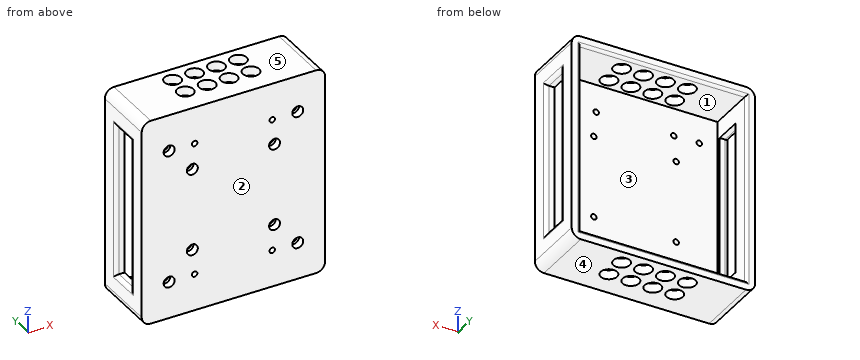
```python
from build123d import *

# Parameters (mm, degrees)
SKETCH1_W            = 100.4
SKETCH1_H            = 113.4
BOSS_EXTRUDE2_DEPTH  = 35
SKETCH2_W            = 90.4
SKETCH2_H            = 103.4
CUT_EXTRUDE1_DEPTH   = 27
FILLET4_R            = 5
SKETCH4_W            = 83.4
SKETCH4_H            = 15
CUT_EXTRUDE3_DEPTH   = 123
FILLET5_R            = 2
FILLET6_R            = 2
SKETCH3_R            = 4.5
CUT_EXTRUDE4_DEPTH   = 123
SKETCH5_R            = 1.5
CUT_EXTRUDE5_DEPTH   = 37
SKETCH6_R            = 3
CUT_EXTRUDE6_DEPTH   = 4
SKETCH7_R            = 1.5
CUT_EXTRUDE7_DEPTH   = 17
SKETCH8_R            = 1.5
CUT_EXTRUDE8_DEPTH   = 9
SKETCH9_R            = 3
CUT_EXTRUDE9_DEPTH   = 4
LPATTERN2_COUNT      = 4
LPATTERN2_PITCH      = 12
LPATTERN2_COUNT_DIR2 = 2
LPATTERN2_PITCH_DIR2 = 12
FILLET7_R            = 1.5


with BuildPart() as part:
    # Sketch1 → Boss-Extrude2 (new body)
    with BuildSketch(Plane(origin=(0, 0, 0), x_dir=(1, 0, 0), z_dir=(0, 1, 0))):
        Rectangle(SKETCH1_W, SKETCH1_H)
    extrude(amount=BOSS_EXTRUDE2_DEPTH)

    # Sketch2 → Cut-Extrude1 (cut)
    with BuildSketch(Plane(origin=(0, 35, 0), x_dir=(1, 0, 0), z_dir=(0, 1, 0))):
        Rectangle(SKETCH2_W, SKETCH2_H)
    extrude(amount=-CUT_EXTRUDE1_DEPTH, mode=Mode.SUBTRACT)

    # Fillet4
    fillet4_edges = [part.edges().sort_by_distance(p)[0] for p in [
        (-50.2, 17.5, 56.7),
        (50.2, 17.5, 56.7),
        (50.2, 17.5, -56.7),
        (-50.2, 17.5, -56.7),
    ]]
    fillet(fillet4_edges, radius=FILLET4_R)

    # Sketch4 → Cut-Extrude3 (cut)
    with BuildSketch(Plane(origin=(50.2, 0, 0), x_dir=(0, 0, -1), z_dir=(1, 0, 0))):
        with Locations((0, 17.5)):
            Rectangle(SKETCH4_W, SKETCH4_H)
    extrude(amount=-CUT_EXTRUDE3_DEPTH, mode=Mode.SUBTRACT)

    # Fillet5
    fillet5_edges = [part.edges().sort_by_distance(p)[0] for p in [
        (50.2, 17.5, 41.7),
        (50.2, 10, 0),
        (50.2, 17.5, -41.7),
        (50.2, 25, 0),
    ]]
    fillet(fillet5_edges, radius=FILLET5_R)

    # Fillet6
    fillet6_edges = [part.edges().sort_by_distance(p)[0] for p in [
        (-50.2, 17.5, 41.7),
        (-50.2, 25, 0),
        (-50.2, 17.5, -41.7),
        (-50.2, 10, 0),
    ]]
    fillet(fillet6_edges, radius=FILLET6_R)

    # Sketch3 → Cut-Extrude4 (cut)
    with BuildSketch(Plane(origin=(0, 0, -56.7), x_dir=(-1, 0, 0), z_dir=(0, 0, -1))):
        with Locations((-18, 14.5)):
            Circle(SKETCH3_R)
    cut_extrude4 = extrude(amount=-CUT_EXTRUDE4_DEPTH, mode=Mode.SUBTRACT)

    # Sketch5 → Cut-Extrude5 (cut)
    with BuildSketch(Plane(origin=(0, 8, 0), x_dir=(1, 0, 0), z_dir=(0, 1, 0))):
        with Locations((-22.5, 22.5)):
            Circle(SKETCH5_R)
        with Locations((22.5, 22.5)):
            Circle(SKETCH5_R)
        with Locations((-22.5, -22.5)):
            Circle(SKETCH5_R)
        with Locations((22.5, -22.5)):
            Circle(SKETCH5_R)
    extrude(amount=-CUT_EXTRUDE5_DEPTH, mode=Mode.SUBTRACT)

    # Sketch6 → Cut-Extrude6 (cut)
    with BuildSketch(Plane.XZ):
        with Locations((-22.5, 22.5)):
            Circle(SKETCH6_R)
        with Locations((-22.5, -22.5)):
            Circle(SKETCH6_R)
        with Locations((22.5, 22.5)):
            Circle(SKETCH6_R)
        with Locations((22.5, -22.5)):
            Circle(SKETCH6_R)
    extrude(amount=-CUT_EXTRUDE6_DEPTH, mode=Mode.SUBTRACT)

    # Sketch7 → Cut-Extrude7 (cut)
    with BuildSketch(Plane.XZ):
        with Locations((-21.25, 36.5)):
            Circle(SKETCH7_R)
        with Locations((-21.25, -36.5)):
            Circle(SKETCH7_R)
        with Locations((21.25, -36.5)):
            Circle(SKETCH7_R)
        with Locations((21.25, 36.5)):
            Circle(SKETCH7_R)
    extrude(amount=-CUT_EXTRUDE7_DEPTH, mode=Mode.SUBTRACT)

    # Sketch8 → Cut-Extrude8 (cut)
    with BuildSketch(Plane(origin=(0, 8, 0), x_dir=(1, 0, 0), z_dir=(0, 1, 0))):
        with Locations((-35.2, 36.6)):
            Circle(SKETCH8_R)
        with Locations((35.2, 36.6)):
            Circle(SKETCH8_R)
        with Locations((-35.2, -36.7)):
            Circle(SKETCH8_R)
        with Locations((35.2, -36.7)):
            Circle(SKETCH8_R)
    extrude(amount=-CUT_EXTRUDE8_DEPTH, mode=Mode.SUBTRACT)

    # Sketch9 → Cut-Extrude9 (cut)
    with BuildSketch(Plane.XZ):
        with Locations((-35.2, 36.7)):
            Circle(SKETCH9_R)
        with Locations((35.2, 36.7)):
            Circle(SKETCH9_R)
        with Locations((-35.2, -36.6)):
            Circle(SKETCH9_R)
        with Locations((35.2, -36.6)):
            Circle(SKETCH9_R)
    extrude(amount=-CUT_EXTRUDE9_DEPTH, mode=Mode.SUBTRACT)

    # LPattern2: Cut-Extrude4 4 × 2
    with Locations(*[(-i * LPATTERN2_PITCH, j * LPATTERN2_PITCH_DIR2, 0) for i in range(LPATTERN2_COUNT) for j in range(LPATTERN2_COUNT_DIR2) if (i, j) != (0, 0)]):
        add(cut_extrude4, mode=Mode.SUBTRACT)

    # Fillet7
    fillet7_edges = [part.edges().sort_by_distance(p)[0] for p in [
        (45.2, 35, 0),
        (0, 35, -51.7),
        (-45.2, 35, 0),
        (0, 35, 51.7),
    ]]
    fillet(fillet7_edges, radius=FILLET7_R)


solid = part.part
```
Check sheet for the modelled part. Datum: model origin and axes. Units: mm. Face numbers are marked on the shaded views. A direction names the side the tool comes from. Give positions to 0.01 mm unless a question says otherwise; leave off trailing zeros. Write each loop counter-clockwise with the first axis right and the second up, starting at its lowest first coordinate (ties: lowest second). Pieces come first, ordered by that corner, then holes.
Item 1: Gauge pin test, flat ends, axial feed: pin 1 (10 mm diameter, centred on y = 16, z = -43, fed in from -X); pin 2 (0.9 mm diameter, centred on x = 46, z = -20, fed in from +Y); pin 3 (1.5 mm diameter, centred on x = -47, y = 16.5, fed in from +Z); pin 4 (5.5 mm diameter, centred on x = -35.2, z = 36.7, fed in from +Y). Record the tip position at first contact, or that the pin passes through.
Item 2: Cross-section at B-B (z = 31). Enter the section's corners in (x, y), and give its area (3 significant figures).
Item 3: Cross-section at A-A (x = -35.2). Enter the section's corners in (y, z).
Item 4: Draft check along Z on the marked faces 3, 4 and 5. Enter one of: released by +Z, released by -Z, zero draft, split by the parting line, or undercut.
Item 5: Access from +Z, -Z, +X, -X, +Y, -Y to the whole of each face (thin tool, end or side, straight path). Record for the marked faces 1 and 2.
Item 6: Cross-section at C-C (x = 18). Enter the section's corners in (y, z), and give its area (3 significant figures).
Item 7: Cross-section at D-D (y = 14.5). Count the separate pieces of the cut face and the enclosed holes in it, and give its area (3 significant figures).
Item 8: Scan lines: L1, parallel to Y at x = -6, z = 53.45; L2, parallel to Z at x = 35.2, y = 2.3; L3, parallel to X at y = 6.3, z = 36.7. Record each from-to range of solid material in increasing order.
Report:
1. pin 1: stops at x = -50.2
1. pin 2: stops at y = 34.98
1. pin 3: stops at z = 56.59
1. pin 4: stops at y = 8
2. outline: (-50.2, 0) - (50.2, 0) - (50.2, 8) arc R2 ccw to (48.2, 10) - (45.2, 10) - (45.2, 8) - (-45.2, 8) - (-45.2, 10) - (-48.2, 10) arc R2 ccw to (-50.2, 8) - close; (-50.2, 27) arc R2 ccw to (-48.2, 25) - (-45.2, 25) - (-45.2, 33.5) arc R1.5 ccw to (-46.7, 35) - (-50.2, 35) - close; (45.2, 25) - (48.2, 25) arc R2 ccw to (50.2, 27) - (50.2, 35) - (46.7, 35) arc R1.5 ccw to (45.2, 33.5) - close
2. area: 919 mm2
3. outline: (0, -56.7) - (35, -56.7) - (35, -53.2) arc R1.5 ccw to (33.5, -51.7) - (8, -51.7) - (8, -38.1) - (4, -38.1) - (4, -39.6) - (0, -39.6) - close; (0, -33.6) - (4, -33.6) - (4, -35.1) - (8, -35.1) - (8, 35.2) - (4, 35.2) - (4, 33.7) - (0, 33.7) - close; (0, 39.7) - (4, 39.7) - (4, 38.2) - (8, 38.2) - (8, 51.7) - (33.5, 51.7) arc R1.5 ccw to (35, 53.2) - (35, 56.7) - (0, 56.7) - close
4. face 3: undercut
4. face 4: released by -Z
4. face 5: released by +Z
5. face 1: +Y
5. face 2: +Z, -Z, +X, -X, -Y
6. outline: (0, -56.7) - (10, -56.7) - (10, -51.7) - (8, -51.7) - (8, 51.7) - (10, 51.7) - (10, 56.7) - (0, 56.7) - close; (19, -56.7) - (22, -56.7) - (22, -51.7) - (19, -51.7) - close; (19, 51.7) - (22, 51.7) - (22, 56.7) - (19, 56.7) - close; (31, -56.7) - (35, -56.7) - (35, -53.2) arc R1.5 ccw to (33.5, -51.7) - (31, -51.7) - close; (31, 51.7) - (33.5, 51.7) arc R1.5 ccw to (35, 53.2) - (35, 56.7) - (31, 56.7) - close
6. area: 996 mm2
7. separate pieces: 10
7. enclosed holes: 0
7. area: 819 mm2
8. L1: y = 0 to 10, 19 to 22, 31 to 35
8. L2: z = -56.7 to -39.6, -33.6 to 33.7, 39.7 to 56.7
8. L3: x = -50.2 to -36.7, -33.7 to -22.74, -19.76 to 19.76, 22.74 to 33.7, 36.7 to 50.2
